CAD build for the part. Positions are in the model's coordinates, mm. A direction names the side the tool comes from. Round coordinates to 2 decimals unless told otherwise and drop trailing zeros. Loops run counter-clockwise (first coordinate to the right, second up) from the corner with the lowest first, then second, coordinate; pieces in that order, holes last.
```python
from build123d import *

# Parameters (mm, degrees)
SKETCH2_R          = 1.5
CUT_EXTRUDE1_DEPTH = 10
SKETCH3_R          = 2
CUT_EXTRUDE2_DEPTH = 26.612497075
CIRPATTERN1_COUNT  = 2
CIRPATTERN1_ANGLE  = 90
CHAMFER1_SIZE      = 1


with BuildPart() as part:
    # Sketch1 → Revolve1 (revolve)
    with BuildSketch(Plane.XY, mode=Mode.PRIVATE) as revolve1_sk:
        Polygon((10, 12), (6.5, 12), (6.5, 5), (5, 5), (5, 0), (16, 0), (16, 3), (10, 5), align=None)
    revolve(revolve1_sk.sketch.rotate(Axis((0, 0, 0), (0, 1, 0)), 90), axis=Axis((0, 0, 0), (0, 1, 0)))

    # Sketch2 → Cut-Extrude1 (cut)
    with BuildSketch(Plane.XZ):
        with Locations(Location((0, 12, 0), (0, 0, 270))):
            Circle(SKETCH2_R)
        with Locations(Location((8.485281374, 8.485281374, 0), (0, 0, 270))):
            Circle(SKETCH2_R)
        with Locations(Location((12, 0, 0), (0, 0, 270))):
            Circle(SKETCH2_R)
        with Locations(Location((8.485281374, -8.485281374, 0), (0, 0, 270))):
            Circle(SKETCH2_R)
        with Locations(Location((0, -12, 0), (0, 0, 270))):
            Circle(SKETCH2_R)
        with Locations(Location((-8.485281374, -8.485281374, 0), (0, 0, 270))):
            Circle(SKETCH2_R)
        with Locations(Location((-12, 0, 0), (0, 0, 270))):
            Circle(SKETCH2_R)
        with Locations(Location((-8.485281374, 8.485281374, 0), (0, 0, 270))):
            Circle(SKETCH2_R)
    extrude(amount=-CUT_EXTRUDE1_DEPTH, mode=Mode.SUBTRACT)

    # Sketch3 → Cut-Extrude2 (cut, through all)
    with BuildSketch(Plane.XY):
        with Locations(Location((0, 8.5, 0), (0, 0, 270.000000001))):
            Circle(SKETCH3_R)
    cut_extrude2 = extrude(amount=-CUT_EXTRUDE2_DEPTH, mode=Mode.SUBTRACT)

    # CirPattern1: Cut-Extrude2 ×2 about axis
    cirpattern1_axis = Axis((0, 12, 0), (0, -1, 0))
    for i in range(1, CIRPATTERN1_COUNT):
        add(cut_extrude2.rotate(cirpattern1_axis, i * CIRPATTERN1_ANGLE / (CIRPATTERN1_COUNT - 1)), mode=Mode.SUBTRACT)

    # Chamfer1
    chamfer1_edges = [part.edges().sort_by_distance(p)[0] for p in [
        (0, 12, 10),
    ]]
    chamfer(chamfer1_edges, length=CHAMFER1_SIZE)


solid = part.part
```
Item 1: Probe line 1 (X direction, y = 2.15, z = 0); line 2 (X direction, y = 2.5, z = 8.5); line 3 (Z direction, x = -1, y = 1.75). List the from-to ranges inside material, lowest first.
Answers follow:
line 1: x = -16 to -13.5, -10.5 to -5, 5 to 10.5, 13.5 to 16
line 2: x = -13.56 to -9.99, -6.99 to 6.99, 9.99 to 13.56
line 3: z = -15.97 to -13.12, -10.88 to -4.9, 4.9 to 10.88, 13.12 to 15.97
Item 2: Two-plate mould, pull along Z, no slides. Class faces 6 (the flat face through (-4, 0, -4)), 7 (the cylindrical face through (-7.47, 2.38, -7.38)), 8 (the cylindrical face through (0, 8, 10)): released by +Z, released by -Z, zero draft, split by the parting line, or undercut.
Answers follow:
face 6: zero draft
face 7: undercut
face 8: split by the parting line
Item 3: Flat gauge pins, fed straight in: P1, Ø4, axis at x = 1.5, z = 3, coming from the +Y side; P2, Ø5, axis at x = 5.5, y = 4, coming from the +Z side; P3, Ø5, axis at y = 8.5, z = 0, coming from the +X side. Where does each tip first touch, or does it go through?
Answers follow:
P1: stops at y = 5
P2: stops at z = 15.67
P3: stops at x = 10
Item 4: Cut at B-B, the plane y = 8.25. Give the cut face in (x, z).
Answers follow:
outline: (-1.98, -9.8) - (-1.98, -6.19) arc R6.5 cw (long way) to (6.19, 1.98) - (9.8, 1.98) arc R10 ccw (long way) to start; (1.98, -9.8) arc R10 ccw to (9.8, -1.98) - (6.19, -1.98) arc R6.5 cw to (1.98, -6.19) - close
Item 5: 3-axis set-ups, long thin cutter, end or side, ignore diameter. For faces 1 (the cylindrical face through (1.983, 8.76, -8.066)), 2 (the flat face through (6, 12, -3)), 3 (the flat face through (5, 5, -2)), 4 (the cylindrical face through (0, 2, 5)), 5 (the cylindrical face through (8.068, 8.76, 1.983)): which of +Z, -Z, +X, -X, +Y, -Y reach the whole face in a straight line?
Answers follow:
face 1: -Z
face 2: +Z, -Z, +X, -X, +Y
face 3: +Y
face 4: +Y, -Y
face 5: +X
Item 6: Cut at A-A, the plane x = 0. State how many separate pieces and enclosed holes the cut face has, plus the area to 3 significant figures.
Answers follow:
separate pieces: 5
enclosed holes: 0
area: 106 mm2
